```python
from build123d import *

# Parameters (mm, degrees)
SKETCH_2_OUTSIDE_W  = 27.09
SKETCH_2_OUTSIDE_H  = 27.09
CUT_EXTRUDE_1_DEPTH = 28.18
CHAMFER_1_SIZE      = 1


with BuildPart() as part:
    # Эскиз1 → Повернуть1 (revolve)
    with BuildSketch(Plane.XY):
        Polygon((-6.58, 0), (-6.58, 8.85), (0, 8.85), (0, 7.448974596), (0.6, 7.288205081), (0.6, 5), (20.6, 5), (20.6, 0), align=None)
    revolve(axis=Axis((-1000, 0, 0), (1, 0, 0)))

    # Эскиз2 outside → Вырез-Вытянуть1 (cut, through all)
    with BuildSketch(Plane.ZY.offset(6.58)):
        Rectangle(SKETCH_2_OUTSIDE_W, SKETCH_2_OUTSIDE_H)
        Polygon((0, -8.85), (7.664324823, -4.425), (7.664324823, 4.425), (0, 8.85), (-7.664324823, 4.425), (-7.664324823, -4.425), align=None, mode=Mode.SUBTRACT)
    extrude(amount=-CUT_EXTRUDE_1_DEPTH, mode=Mode.SUBTRACT)

    # Эскиз4 → Вырез-Повернуть1 (revolve, cut)
    with BuildSketch(Plane.XY):
        Polygon((-6.58, 8.075), (-6.297923068, 8.85), (-6.58, 8.85), align=None)
    revolve(axis=Axis((-1000, 0, 0), (1, 0, 0)), mode=Mode.SUBTRACT)

    # Фаска1
    chamfer_1_edges = [part.edges().sort_by_distance(p)[0] for p in [
        (20.6, -5, 0),
    ]]
    chamfer(chamfer_1_edges, length=CHAMFER_1_SIZE)


solid = part.part
```
Part model, mm, in its own coordinate system. A direction names the side the tool comes from. Give positions to 0.01 mm unless a question says otherwise; leave off trailing zeros. Write each loop counter-clockwise with the first axis right and the second up, starting at its lowest first coordinate (ties: lowest second). Pieces come first, ordered by that corner, then holes. Notation, with made-up numbers: (79, 4.25) -> (104, 4.25) arc R22 cw to (104, 41.25) -> close; hole circle Ø9 at (83, 83.5). An arc over 180 degrees is marked (long way). Put each result on its own line as item: value. Start each with the question number.
Item 1: Wall check: L1, parallel to Y at x = 6.25, z = 0.25; L2, parallel to X at y = 5.25, z = 2.5; L3, parallel to Z at x = 13.5, y = 2.75. Give the ranges that are in metal, low to high. Write a range as [from, to].
Item 2: Which spindle directions (+Z, -Z, +X, -X, +Y, -Y) get a long thin tool onto all of the face, cutting with end or side? Do faces 1 (the face through (-3, 0, -7.664)), 2 (the face through (0.6, -2, -5)). Say none if no direction does.
Item 3: Cut at A-A (y = 0). List the corners of the cut face in (x, z), then the cut area to 3 significant figures.
Item 4: Cut at B-B (x = -3.75). List the corners of the cut face in (y, z) (3 decimals), then the cut area to 3 significant figures.
Item 5: Pin check, flat tips, straight feed: pin 1 Ø8 at (x, y) = (11.5, -4.5) entering from +Z; pin 2 Ø10 at (x, y) = (8.5, -4.5) entering from -Z; pin 3 Ø3 at (x, z) = (16.5, -1) entering from -Y. Stop position of each tip, or through.
Item 6: Cut at C-C (x = 11). List the corners of the cut face in (y, z).
Answer list:
1. L1: y = [-4.99, 4.99]
1. L2: x = [-6.58, 0.6]
1. L3: z = [-4.18, 4.18]
2. face 1: -Z, +X, -X, +Y, -Y
2. face 2: +X
3. outline: (-6.58, -7.66) -> (0, -7.66) -> (0, -7.45) -> (0.6, -7.29) -> (0.6, -5) -> (19.6, -5) -> (20.6, -4) -> (20.6, 4) -> (19.6, 5) -> (0.6, 5) -> (0.6, 7.29) -> (0, 7.45) -> (0, 7.66) -> (-6.58, 7.66) -> close
3. area: 309 mm2
4. outline: (-8.85, 0) -> (-4.425, -7.664) -> (4.425, -7.664) -> (8.85, 0) -> (4.425, 7.664) -> (-4.425, 7.664) -> close
4. area: 203 mm2
5. pin 1: stops at z = 4.97
5. pin 2: stops at z = -5
5. pin 3: stops at y = -5
6. outline: circle Ø10 at (0, 0)
